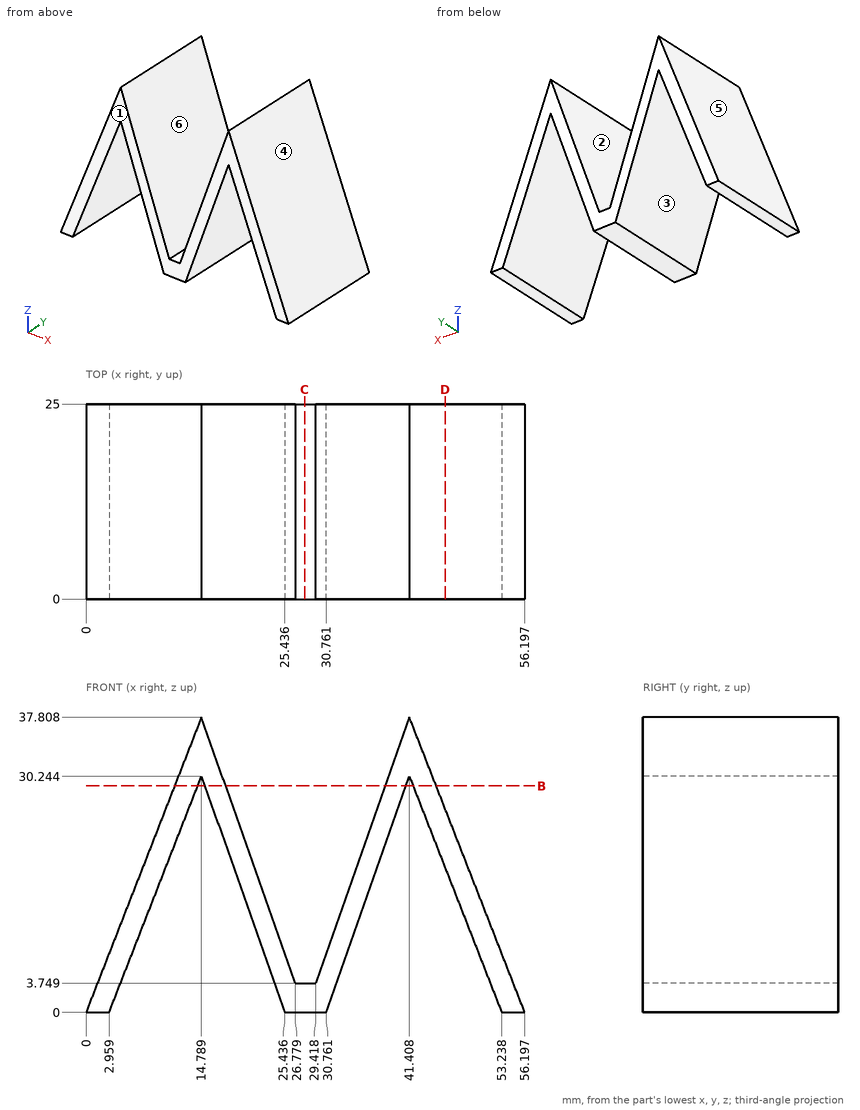
Could you check a few things on this drawing? It's one solid part, dimensions in mm from its lowest x, y, z. A direction names the side the tool comes from. Coordinates: 2 decimals unless noted, no trailing zeros. Order: outer loops, then holes, each group sorted by start corner. A loop starts at its lowest first (then second) coordinate and runs counter-clockwise, first axis right, second up. Notation, with made-up numbers: (52.5, 11) - (106.5, 11) arc R21 ccw to (106.5, 28) - close; hole circle Ø11 at (-12.5, -17.5). An arc over 180 degrees is marked (long way). Answer as a JSON object with one key per item and string values. Group by question number.
Q1. I need wall thicknesses on line 1 (X direction, y = 7.75, z = 13) (1 decimal); line 2 (X direction, y = 7.75, z = 18) (1 decimal); line 3 (X direction, y = 1.5, z = 3.5) (1 decimal). Which ranges of each line are inside material? Lowest first, please. Write a range as from..to.
Q2. Imagine slicing it at B-B (z = 29). Please give me the cut outline in (x, y) (1 decimal).
Q3. On a 3-axis mill with a long thin cutter (end or side, diameter ignored), from which of +Z, -Z, +X, -X, +Y, -Y can I reach the whole of each face in a straight line? I mean the marked faces 1, 2 and 3. Say none if no direction works.
Q4. We'd pull the mould along X, two halves only. Please class the marked faces 4, 5 and 6: +X half, -X half, draft (parallel to the pull), parting line (faces both ways), or undercut.
Q5. Will these pins go through, and if not, where does the flat tip stop? P1, Ø5, axis at x = 30, z = 10.5, coming from the -Y side; P2, Ø1.5, axis at y = 22.5, z = 22.5, coming from the +X side; P3, Ø8, axis at y = 13, z = 13, coming from the +X side; P4, Ø2, axis at y = 21, z = 6, coming from the -X side (1 decimal).
Q6. Imagine slicing it at C-C (x = 28). Please give me the cut outline in (y, z).
Q7. Imagine slicing it at D-D (x = 46). Please give me the cut outline in (y, z) (1 decimal).
Determined:
{
 "1": {"line 1": "x = 5.1..8, 20.9..23.5, 32.7..35.3, 48.2..51.1", "line 2": "x = 7..10, 19.1..21.8, 34.4..37.1, 46.2..49.2", "line 3": "x = 1.4..4.3, 24.2..32, 51.9..54.8"},
 "2": {"outline": "(11.3, 0) - (14.3, 0) - (14.3, 25) - (11.3, 25) - close; (15.2, 0) - (17.9, 0) - (17.9, 25) - (15.2, 25) - close; (38.3, 0) - (41, 0) - (41, 25) - (38.3, 25) - close; (41.9, 0) - (44.9, 0) - (44.9, 25) - (41.9, 25) - close"},
 "3": {"face 1": "+Z, -Z, +X, -X, -Y", "face 2": "+Z, +Y, -Y", "face 3": "-Z, +Y, -Y"},
 "4": {"face 4": "+X half", "face 5": "-X half", "face 6": "undercut"},
 "5": {"P1": "stops at y = 0", "P2": "stops at x = 47.69", "P3": "stops at x = 52.68", "P4": "stops at x = 2"},
 "6": {"outline": "(0, 0) - (25, 0) - (25, 3.75) - (0, 3.75) - close"},
 "7": {"outline": "(0, 18.5) - (25, 18.5) - (25, 26.1) - (0, 26.1) - close"}
}
